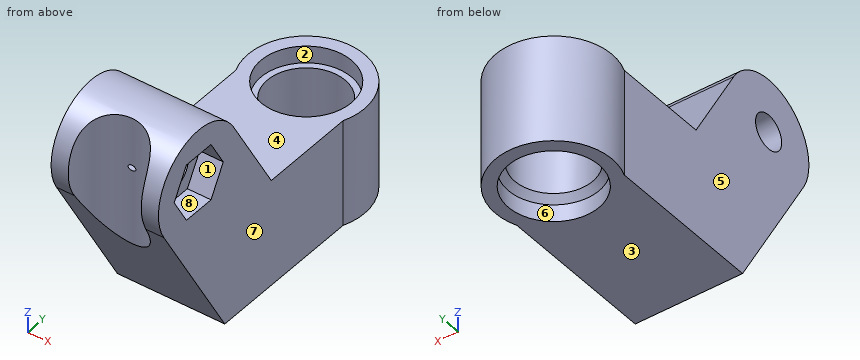
Autodesk Inventor part; units mm, degrees
ref_plane "YZ Plane" through (0, 0, 0) normal (1, 0, 0) x (0, 1, 0)
ref_plane "XZ Plane" through (0, 0, 0) normal (0, 1, 0) x (-1, 0, 0)
ref_plane "XY Plane" through (0, 0, 0) normal (0, 0, 1) x (1, 0, 0)
sketch "Sketch1" plane through (0, 0, 0) normal (1, 0, 0) x (0, 1, 0)
  circle A0 centre (-50, 14) radius 4.05
  arc A1 (-39.1747, 20.25) -> (-60.8253, 7.75) centre (-50, 14) ccw
  line L0 (0, 0) -> (0, -25)
  line L1 (0, -25) -> (-41.9171, -25)
  line L2 (-41.9171, -25) -> (-60.8253, 7.75)
  line L3 (0, 0) -> (-27.4833, 0)
  line L4 (-27.4833, 0) -> (-39.1747, 20.25)
  dimension "d0" = 8.1
  dimension "d2" = 50
  dimension "d3" = 14
  dimension "d4" = 25
  dimension "d6" = 25
  dimension "d40" = 120
extrude "Extrusion1" add sketch "Sketch1" along normal mid plane 25
sketch "Sketch2" plane through (-12.5, -27.4833, 0) normal (0, 0, 1) x (1, 0, 0)
  circle A0 centre (12.5, 27.4833) radius 12.5
extrude "Extrusion2" add sketch "Sketch2" against normal up to surface (25 mm away)
sketch "Sketch13" plane through (-12.5, -27.4833, 0) normal (0, 0, 1) x (1, 0, 0)
  arc A0 (25, 27.4833) -> (0, 27.4833) centre (12.5, 27.4833) ccw
  circle A1 centre (12.5, 27.4833) radius 9.05
  dimension "d59" = 18.1
extrude "Extrusion13" cut sketch "Sketch13" against normal through all
sketch "Sketch14" plane through (-12.5, -27.4833, 0) normal (0, 0, 1) x (1, 0, 0)
  circle A0 centre (12.5, 27.4833) radius 9.05
  arc A1 (25, 27.4833) -> (0, 27.4833) centre (12.5, 27.4833) ccw
  circle A2 centre (12.5, 27.4833) radius 10.55
  dimension "d63" = 21.1
extrude "Extrusion14" cut sketch "Sketch14" against normal blind 4
sketch "Sketch15" plane through (12.5, -41.9171, -25) normal (0, 0, -1) x (-1, 0, 0)
  circle A0 centre (12.5, 41.9171) radius 9.05
  arc A1 (25, 41.9171) -> (0, 41.9171) centre (12.5, 41.9171) ccw
  circle A2 centre (12.5, 41.9171) radius 10.55
  dimension "d67" = 21.1
extrude "Extrusion15" cut sketch "Sketch15" against normal blind 4
chamfer "Chamfer4" distance 1.5 angle 45 1 edges at (-9.05, 0, -21)
sketch "Sketch16" plane through (-12.5, -27.4833, 0) normal (0, 0, 1) x (1, 0, 0)
  circle A0 centre (12.5, 27.4833) radius 10.55
  arc A1 (25, 27.4833) -> (0, 27.4833) centre (12.5, 27.4833) ccw
  circle A2 centre (12.5, 27.4833) radius 13.55
  dimension "d76" = 3
extrude "Extrusion16" add sketch "Sketch16" against normal up to surface (25 mm away)
sketch "Sketch17" plane through (12.5, 0, 0) normal (1, 0, 0) x (0, 0, -1)
  arc A0 (-19.5, -40.4737) -> (-8.5, -59.5263) centre (-14, -50) ccw
  line L0 (-14, -42.379) -> (-7.4, -46.1895)
  line L1 (-7.4, -46.1895) -> (-7.4, -53.8105)
  line L2 (-7.4, -53.8105) -> (-14, -57.621)
  line L3 (-14, -57.621) -> (-20.6, -53.8105)
  line L4 (-20.6, -53.8105) -> (-20.6, -46.1895)
  line L5 (-20.6, -46.1895) -> (-14, -42.379)
  point P0 (0, 0)
  dimension "d80" = 13.2
extrude "Extrusion17" cut sketch "Sketch17" against normal blind 5.5
sketch "Sketch18" plane through (12.5, -41.9171, -25) normal (0, 0, -1) x (-1, 0, 0)
  line L0 (25, -20.5829) -> (0, -20.5829)
  circle A0 centre (12.5, -20.5829) radius 8.5
  dimension "d83" = 17
extrude "Extrusion18" cut sketch "Sketch18" against normal through all
properties part number "hub top"
Model file for the job. Use its own axes, mm. Face numbers are marked on the shaded views. A direction names the side the tool comes from. Coordinates: 2 decimals unless noted, no trailing zeros. Write each loop counter-clockwise with the first axis right and the second up, starting at its lowest first coordinate (ties: lowest second). Pieces come first, ordered by that corner, then holes. Notation, with made-up numbers: (-19.75, 52) -> (39.25, 52) arc R6 ccw to (39.25, 59) -> close; hole circle Ø6 at (78, 58). An arc over 180 degrees is marked (long way). One line per item, written item: value. Start each with the question number.
1) Slice it at C-C on z = -14. Write the cut outline in (x, y).
2) Slice it at A-A on y = -50. Write the cut outline in (x, z), then the cut area to 3 significant figures.
3) Probe probe 1 along Y at (x, z) = (0, -1.95); probe 2 along X at (y, z) = (-34, -19); probe 3 along Z at (x, y) = (-5, -22). List the from-to ranges inside material, lowest first.
4) Slice it at D-D on z = 19. Write the cut outline in (x, y).
5) Pull direction Z, two halves, no side cores. Call the marked faces 1, 2 and 3: +Z half, -Z half, draft (parallel to the pull), parting line (faces both ways), or undercut.
6) Which spindle directions (+Z, -Z, +X, -X, +Y, -Y) get a long thin tool onto all of the face, cutting with end or side? Do the marked faces 4, 5, 6, 7 and 8. Say none if no direction does.
7) Flat gauge pins, fed straight in: pin 1 Ø13 at (y, z) = (-50, 14) entering from -X; pin 2 Ø2 at (y, z) = (-7, -4.5) entering from +X; pin 3 Ø6 at (x, y) = (9.5, -49) entering from -Z. Where does each tip first touch, or does it go through?
Answers follow:
1. outline: (-12.5, -48.27) -> (12.5, -48.27) -> (12.5, -5.23) arc R13.55 ccw (long way) to (-12.5, -5.23) -> close; hole circle Ø18.1 at (0, 0)
2. outline: (-12.5, -11) -> (12.5, -11) -> (12.5, 7.4) -> (7, 7.4) -> (7, 9.95) -> (-12.5, 9.95) -> close; (-12.5, 18.05) -> (7, 18.05) -> (7, 20.6) -> (12.5, 20.6) -> (12.5, 26.5) -> (-12.5, 26.5) -> close
2. area: 707 mm2
3. probe 1: -54 to -10.55, 10.55 to 13.55
3. probe 2: -12.5 to 12.5
3. probe 3: -25 to 0
4. outline: (-12.5, -61.46) -> (-8.44, -61.46) arc R8.5 cw to (8.44, -61.46) -> (12.5, -61.46) -> (12.5, -54.73) -> (7, -54.73) -> (7, -45.27) -> (12.5, -45.27) -> (12.5, -38.45) -> (-12.5, -38.45) -> close
5. face 1: undercut
5. face 2: draft
5. face 3: -Z half
6. face 4: +Z, +X, -X, +Y
6. face 5: +Z, -Z, -X, -Y
6. face 6: -Z
6. face 7: +Z, -Z, +X, -Y
6. face 8: +X
7. pin 1: x = -12.5
7. pin 2: x = 12.5
7. pin 3: z = -17.93
